Design review of the part built by this model. Coordinates are the model's own, in mm. Face numbers are marked on the shaded views. Coordinates: 2 decimals unless noted, no trailing zeros. Loops run counter-clockwise (first coordinate to the right, second up) from the corner with the lowest first, then second, coordinate; pieces in that order, holes last. Notation, with made-up numbers: M 44,14.5 L 76,14.5 A34 ccw 76,45.5 Z; hole C -36.75,-8.5 d5. An arc over 180 degrees is marked long. Put each result on its own line as item: value. Start each with the question number.
(1) For probe 1 along X at (y, z) = (20, 0); probe 2 along X at (y, z) = (9, 9); probe 3 along Y at (x, z) = (6.5, -8), list the stretches that pass through material, from the lowest coordinate up. Write a range as [from, to].
(2) The part is to be moulded in two halves that separate along X. For the marked faces 1, 2 and 3, say which applies: +X half, -X half, draft (parallel to the pull), parting line (faces both ways), or undercut.
(3) Take a section at A-A, the plane y = 14. Give the boundary of the cut face in (x, z), then the cut area to 3 significant figures.
(4) Clearance check with flat-ended pins moving along their axes: pin 1 (8 mm diameter, centred on x = -3, z = 1, fed in from +Y); pin 2 (4 mm diameter, centred on x = -10, y = 7.5, fed in from -Z); pin 3 (1 mm diameter, centred on y = 22.5, z = 1.5, fed in from -X). State where each tip first meets the part, or that it passes through.
(5) Take a section at B-B, the plane z = 0. Give the boundary of the cut face in (x, y).
```python
from build123d import *

# Parameters (mm, degrees)
SKETCH1_R           = 17
BOSS_EXTRUDE1_DEPTH = 4
SKETCH2_R           = 17
SKETCH2_R_2         = 13.5
BOSS_EXTRUDE2_DEPTH = 26.5
FILLET1_R           = 2


with BuildPart() as part:
    # Sketch1 → Boss-Extrude1 (new body)
    with BuildSketch(Plane(origin=(0, 0, 0), x_dir=(1, 0, 0), z_dir=(0, 1, 0))):
        with Locations(Location((0, 0, 0), (0, 0, 270))):
            Circle(SKETCH1_R)
    extrude(amount=BOSS_EXTRUDE1_DEPTH)

    # Sketch2 → Boss-Extrude2 (add)
    with BuildSketch(Plane(origin=(0, 4, 0), x_dir=(1, 0, 0), z_dir=(0, 1, 0))):
        with Locations(Location((0, 0, 0), (0, 0, 270))):
            Circle(SKETCH2_R)
        with Locations(Location((0, 0, 0), (0, 0, 270))):
            Circle(SKETCH2_R_2, mode=Mode.SUBTRACT)
    extrude(amount=BOSS_EXTRUDE2_DEPTH)

    # Fillet1
    fillet1_edges = [part.edges().sort_by_distance(p)[0] for p in [
        (0, 0, -17),
        (0, 30.5, -17),
    ]]
    fillet(fillet1_edges, radius=FILLET1_R)


solid = part.part
```
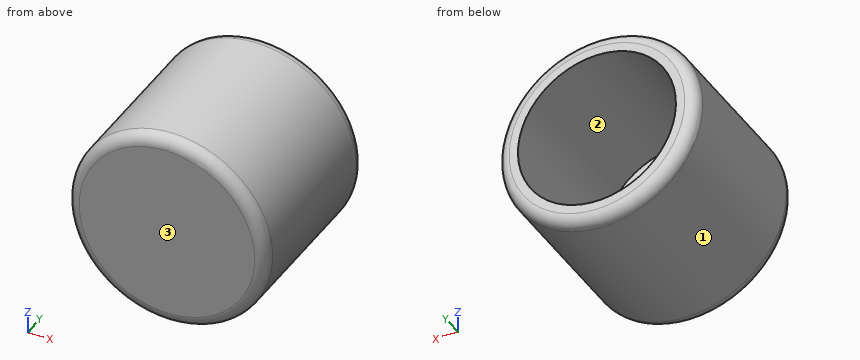
Computed values:
1. probe 1: x = [-17, -13.5], [13.5, 17]
1. probe 2: x = [-14.42, -10.06], [10.06, 14.42]
1. probe 3: y = [0, 4]
2. face 1: parting line
2. face 2: undercut
2. face 3: draft
3. outline: C 0,0 d34; hole C 0,0 d27
3. area: 335 mm^2
4. pin 1: stops at y = 4
4. pin 2: stops at z = -15
4. pin 3: stops at x = -16.97
5. outline: M -17,2 A2 ccw -15,0 L 15,0 A2 ccw 17,2 L 17,28.5 A2 ccw 15,30.5 L 13.5,30.5 L 13.5,4 L -13.5,4 L -13.5,30.5 L -15,30.5 A2 ccw -17,28.5 Z
